Design review of the part built by this model. Coordinates are the model's own, in mm. A direction names the side the tool comes from. Coordinates: 2 decimals unless noted, no trailing zeros. Order: outer loops, then holes, each group sorted by start corner. A loop starts at its lowest first (then second) coordinate and runs counter-clockwise, first axis right, second up. Notation, with made-up numbers: (51.5, 3) -> (102.5, 3) arc R28 ccw to (102.5, 26) -> close; hole circle Ø8 at (86, -21). An arc over 180 degrees is marked (long way). Use a Markdown table: item, result. Add a question column.
Q1. Machinability: for faces 4 (the face through (100, 10, 70)), 5 (the face through (100, 0, 20)), 6 (the face through (-1, -10, -2)), 7 (the face through (-100, -10, 10)), which of the approach directions +Z, -Z, +X, -X, +Y, -Y give a long, thin tool a straight path to every point of the face, cutting with its end or side? Answer none if there is none.
Q2. Add section A-A (z = 38.5). State the section outline as (x, y) points.
Q3. The part is to be moulded in two halves that separate along Z. For faces 1 (the face through (-100, 10, 10)), 2 (the face through (95, 0, 44)), 3 (the face through (-1, -3, -5)), say which applies: pulls with the +Z half, pulls with the -Z half, needs draft (parallel to the pull), parting line crosses it, or undercut.
Q4. Wall thickness on probe 1 along X at (y, z) = (-7.75, 44); probe 2 along Z at (x, y) = (8, -3.75); probe 3 along Z at (x, y) = (-94, 3): over which ranges is each line inside the solid? List them lowest first.
Q5. Add section D-D (y = -7.5). State the section outline as (x, z) points.
Q6. Add section B-B (y = 12.5). State the section outline as (x, z) points, then the cut area to 3 significant figures.
Q7. Add section C-C (z = 69). State the section outline as (x, y) points, then the cut area to 3 significant figures.
Q8. Insertion check: pin 1 (16 mm diameter, centred on x = 0, y = 0, fed in from +Z); pin 2 (3 mm diameter, centred on y = -6, z = 77, fed in from -X); pin 3 (1 mm diameter, centred on x = -46.5, y = 0, fed in from +Z). Each pin has a flat end and moves straight along its axis. Give the tip position at first contact, or say it passes through.
from build123d import *

# Parameters (mm, degrees)
F0_R     = 5
F2_DEPTH = 5
F3_DEPTH = 95
F1_W     = 20
F1_H     = 20
F4_DEPTH = 200
F5_DEPTH = 20


with BuildPart() as f2:
    # F0 (on Top) → F2 (new body)
    with BuildSketch(Plane.XY):
        Polygon((-95, -10), (-95, 10), (-95, 15), (-105, 15), (-105, -15), (-95, -15), align=None)
        with BuildLine():
            ThreePointArc((0, -10), (-10, 0), (0, 10))
            Line((0, 10), (-95, 10))
            Line((-95, 10), (-95, -10))
            Line((-95, -10), (0, -10))
        make_face()
        with BuildLine():
            ThreePointArc((0, 10), (7.071068, 7.071068), (10, 0))
            ThreePointArc((10, 0), (7.071068, -7.071068), (0, -10))
            Line((0, -10), (95, -10))
            Line((95, -10), (95, 10))
            Line((95, 10), (0, 10))
        make_face()
        Polygon((95, 15), (95, 10), (95, -10), (95, -15), (105, -15), (105, 15), align=None)
        with BuildLine():
            ThreePointArc((0, -10), (7.071068, -7.071068), (10, 0))
            ThreePointArc((10, 0), (7.071068, 7.071068), (0, 10))
            ThreePointArc((0, 10), (-10, 0), (0, -10))
        make_face()
        Circle(F0_R, mode=Mode.SUBTRACT)
        Circle(F0_R)
    extrude(amount=-F2_DEPTH)

    # F0 (on Top) → F3 (join)
    with BuildSketch(Plane.XY):
        Polygon((-95, -10), (-95, 10), (-95, 15), (-105, 15), (-105, -15), (-95, -15), align=None)
        Polygon((95, 15), (95, 10), (95, -10), (95, -15), (105, -15), (105, 15), align=None)
    extrude(amount=F3_DEPTH)

    # F1 (on Right) → F4 (cut, symmetric)
    with BuildSketch(Plane.YZ):
        with Locations((0, 10)):
            Rectangle(F1_W, F1_H)
        with Locations((0, 70)):
            Rectangle(F1_W, F1_H)
    extrude(amount=F4_DEPTH, both=True, mode=Mode.SUBTRACT)

    # F0 (on Top) → F5 (join)
    with BuildSketch(Plane.XY):
        with BuildLine():
            ThreePointArc((0, -10), (7.071068, -7.071068), (10, 0))
            ThreePointArc((10, 0), (7.071068, 7.071068), (0, 10))
            ThreePointArc((0, 10), (-10, 0), (0, -10))
        make_face()
        Circle(F0_R, mode=Mode.SUBTRACT)
    extrude(amount=F5_DEPTH)


solid = f2.part
Established:
| question | item | result |
|---|---|---|
| 1 | face 4 | +X, -X |
| 1 | face 5 | +X |
| 1 | face 6 | +Z, -Z, -Y |
| 1 | face 7 | -X |
| 2 | outline | (-105, -15) -> (-95, -15) -> (-95, 15) -> (-105, 15) -> close; (95, -15) -> (105, -15) -> (105, 15) -> (95, 15) -> close |
| 3 | face 1 | undercut |
| 3 | face 2 | needs draft |
| 3 | face 3 | pulls with the -Z half |
| 4 | probe 1 | -105 to -95, 95 to 105 |
| 4 | probe 2 | -5 to 20 |
| 4 | probe 3 | -5 to 0 |
| 5 | outline | (-105, -5) -> (105, -5) -> (105, 0) -> (6.61, 0) -> (6.61, 20) -> (-6.61, 20) -> (-6.61, 0) -> (-105, 0) -> close; (-105, 20) -> (-95, 20) -> (-95, 60) -> (-105, 60) -> close; (-105, 80) -> (-95, 80) -> (-95, 95) -> (-105, 95) -> close; (95, 20) -> (105, 20) -> (105, 60) -> (95, 60) -> close; (95, 80) -> (105, 80) -> (105, 95) -> (95, 95) -> close |
| 6 | outline | (-105, -5) -> (-95, -5) -> (-95, 95) -> (-105, 95) -> close; (95, -5) -> (105, -5) -> (105, 95) -> (95, 95) -> close |
| 6 | area | 2,000 mm^2 |
| 7 | outline | (-105, -15) -> (-95, -15) -> (-95, -10) -> (-105, -10) -> close; (-105, 10) -> (-95, 10) -> (-95, 15) -> (-105, 15) -> close; (95, -15) -> (105, -15) -> (105, -10) -> (95, -10) -> close; (95, 10) -> (105, 10) -> (105, 15) -> (95, 15) -> close |
| 7 | area | 200 mm^2 |
| 8 | pin 1 | z = 20 |
| 8 | pin 2 | through |
| 8 | pin 3 | z = 0 |
